from build123d import *

# Parameters (mm, degrees)
BOSS_EXTRUDE1_DEPTH     = 23
BOSS_EXTRUDE2_DEPTH     = 3
CUT_EXTRUDE1_DEPTH      = 143.828568571
CUT_EXTRUDE1_DEPTH_BACK = 143.828568571
SKETCH4_R               = 1.6
CUT_EXTRUDE2_DEPTH      = 1.5
SKETCH6_W               = 75
SKETCH6_H               = 20
CUT_EXTRUDE4_DEPTH      = 5
SKETCH8_R               = 1.25
SKETCH8_W               = 31.4
SKETCH8_H               = 20
CUT_EXTRUDE5_DEPTH      = 5
SKETCH9_W               = 2
SKETCH9_H               = 4.5
BOSS_EXTRUDE3_DEPTH     = 10
FILLET2_R               = 1
SKETCH10_W              = 12.12
SKETCH10_H              = 31
BOSS_EXTRUDE4_DEPTH     = 2.6
FILLET3_R               = 2
FILLET5_R               = 2
SKETCH11_W              = 2
SKETCH11_H              = 24
BOSS_EXTRUDE5_DEPTH     = 4
FILLET6_R               = 1
FILLET7_R               = 1
SKETCH12_W              = 10.12
SKETCH12_H              = 2
BOSS_EXTRUDE6_DEPTH     = 0.75
FILLET3_OF_MIRROR1_R    = 2
FILLET5_OF_MIRROR1_R    = 2
FILLET6_OF_MIRROR1_R    = 1
FILLET7_OF_MIRROR1_R    = 1


with BuildPart() as part:
    # Sketch1 → Boss-Extrude1 (new body)
    with BuildSketch(Plane(origin=(0, 0, 0), x_dir=(1, 0, 0), z_dir=(0, 1, 0))):
        with BuildLine():
            Line((12.5, 0), (87.5, 0))
            ThreePointArc((87.5, 0), (96.338834765, 3.661165235), (100, 12.5))
            Line((100, 12.5), (100, 87.5))
            ThreePointArc((100, 87.5), (96.338834765, 96.338834765), (87.5, 100))
            Line((87.5, 100), (12.5, 100))
            ThreePointArc((12.5, 100), (3.661165235, 96.338834765), (0, 87.5))
            Line((0, 87.5), (0, 12.5))
            ThreePointArc((0, 12.5), (3.661165235, 3.661165235), (12.5, 0))
        make_face()
        with BuildLine():
            Line((15, 97.5), (85, 97.5))
            ThreePointArc((85, 97.5), (93.838834765, 93.838834765), (97.5, 85))
            Line((97.5, 85), (97.5, 15))
            ThreePointArc((97.5, 15), (93.838834765, 6.161165235), (85, 2.5))
            Line((85, 2.5), (15, 2.5))
            ThreePointArc((15, 2.5), (6.161165235, 6.161165235), (2.5, 15))
            Line((2.5, 15), (2.5, 85))
            ThreePointArc((2.5, 85), (6.161165235, 93.838834765), (15, 97.5))
        make_face(mode=Mode.SUBTRACT)
    extrude(amount=BOSS_EXTRUDE1_DEPTH)

    # Sketch1<2> → Boss-Extrude2 (add)
    with BuildSketch(Plane(origin=(0, 0, 0), x_dir=(1, 0, 0), z_dir=(0, 1, 0))):
        with BuildLine():
            Line((15, 97.5), (85, 97.5))
            ThreePointArc((85, 97.5), (93.838834765, 93.838834765), (97.5, 85))
            Line((97.5, 85), (97.5, 15))
            ThreePointArc((97.5, 15), (93.838834765, 6.161165235), (85, 2.5))
            Line((85, 2.5), (15, 2.5))
            ThreePointArc((15, 2.5), (6.161165235, 6.161165235), (2.5, 15))
            Line((2.5, 15), (2.5, 85))
            ThreePointArc((2.5, 85), (6.161165235, 93.838834765), (15, 97.5))
        make_face()
    extrude(amount=BOSS_EXTRUDE2_DEPTH)

    # Sketch4 → Cut-Extrude1 (cut, two sides: drawn at the far end of the back side and taken through both)
    with BuildSketch(Plane(origin=(0, 3, 0), x_dir=(1, 0, 0), z_dir=(0, 1, 0)).offset(-CUT_EXTRUDE1_DEPTH_BACK)):
        with Locations(Location((88.890872965, 11.109127035, 0), (0, 0, 270))):
            Circle(SKETCH4_R)
        with Locations(Location((11.109127035, 88.890872965, 0), (0, 0, 270))):
            Circle(SKETCH4_R)
    extrude(amount=CUT_EXTRUDE1_DEPTH + CUT_EXTRUDE1_DEPTH_BACK, mode=Mode.SUBTRACT)

    # Sketch5 → Cut-Extrude2 (cut)
    with BuildSketch(Plane(origin=(0, 3, 0), x_dir=(1, 0, 0), z_dir=(0, 1, 0))):
        with BuildLine():
            Line((82.5, 4), (12.5, 4))
            ThreePointArc((12.5, 4), (8.964466094, 5.464466094), (7.5, 9))
            Line((7.5, 9), (7.5, 44))
            Line((7.5, 44), (82.5, 44))
            Line((82.5, 44), (82.5, 4))
        make_face()
    extrude(amount=-CUT_EXTRUDE2_DEPTH, mode=Mode.SUBTRACT)

    # Sketch6 → Cut-Extrude4 (cut)
    with BuildSketch(Plane.XY):
        with Locations((50, 13)):
            Rectangle(SKETCH6_W, SKETCH6_H)
    extrude(amount=-CUT_EXTRUDE4_DEPTH, mode=Mode.SUBTRACT)

    # Sketch8 → Cut-Extrude5 (cut)
    with BuildSketch(Plane(origin=(100, 0, 0), x_dir=(0, 0, -1), z_dir=(1, 0, 0))):
        with Locations((15.15, 11.76333723)):
            Circle(SKETCH8_R)
        with Locations(Location((51.25, 11.76333723, 0), (0, 0, 180))):
            Circle(SKETCH8_R)
        with Locations((33.2, 13)):
            Rectangle(SKETCH8_W, SKETCH8_H)
    extrude(amount=-CUT_EXTRUDE5_DEPTH, mode=Mode.SUBTRACT)

    # Sketch9 → Boss-Extrude3 (add)
    with BuildSketch(Plane.ZY):
        with Locations((-56.5, 11.5)):
            Rectangle(SKETCH9_W, SKETCH9_H)
    extrude(amount=BOSS_EXTRUDE3_DEPTH)

    # Fillet2
    fillet2_edges = [part.edges().sort_by_distance(p)[0] for p in [
        (0, 11.5, -57.5),
        (-5, 13.75, -57.5),
        (0, 9.25, -56.5),
        (-5, 9.25, -57.5),
        (0, 11.5, -55.5),
        (-5, 9.25, -55.5),
        (0, 13.75, -56.5),
        (-5, 13.75, -55.5),
        (-10, 11.5, -57.5),
        (-10, 9.25, -56.5),
        (-10, 11.5, -55.5),
        (-10, 13.75, -56.5),
    ]]
    fillet(fillet2_edges, radius=FILLET2_R - 0.0001)  # a hair under: the kernel refuses the full size

    # Sketch10 → Boss-Extrude4 (add)
    with BuildSketch(Plane(origin=(0, 0, 0), x_dir=(1, 0, 0), z_dir=(0, 1, 0))):
        with Locations((-6.06, 70)):
            Rectangle(SKETCH10_W, SKETCH10_H)
    boss_extrude4 = extrude(amount=BOSS_EXTRUDE4_DEPTH)

    # Fillet3
    fillet3_edges = [part.edges().sort_by_distance(p)[0] for p in [
        (0, 1.3, -54.5),
    ]]
    fillet(fillet3_edges, radius=FILLET3_R)

    # Fillet5
    fillet5_edges = [part.edges().sort_by_distance(p)[0] for p in [
        (0, 1.3, -85.5),
    ]]
    fillet(fillet5_edges, radius=FILLET5_R - 0.0001)  # a hair under: the kernel refuses the full size

    # Sketch11 → Boss-Extrude5 (add)
    with BuildSketch(Plane(origin=(0, 2.6, 0), x_dir=(1, 0, 0), z_dir=(0, 1, 0))):
        with Locations((-11.12, 73.5)):
            Rectangle(SKETCH11_W, SKETCH11_H)
    boss_extrude5 = extrude(amount=BOSS_EXTRUDE5_DEPTH)

    # Fillet6
    fillet6_edges = [part.edges().sort_by_distance(p)[0] for p in [
        (-12.12, 6.6, -73.5),
    ]]
    fillet(fillet6_edges, radius=FILLET6_R)

    # Fillet7
    fillet7_edges = [part.edges().sort_by_distance(p)[0] for p in [
        (-10.12, 2.6, -73.5),
    ]]
    fillet(fillet7_edges, radius=FILLET7_R)

    # Sketch12 → Boss-Extrude6 (add)
    with BuildSketch(Plane(origin=(0, 2.6, 0), x_dir=(1, 0, 0), z_dir=(0, 1, 0))):
        with Locations((-7.06, 55.5)):
            Rectangle(SKETCH12_W, SKETCH12_H)
    boss_extrude6 = extrude(amount=BOSS_EXTRUDE6_DEPTH)

    # Mirror1: Boss-Extrude4, Boss-Extrude5, Boss-Extrude6 across plane
    add(boss_extrude4.mirror(Plane.ZX.offset(11.5)))
    add(boss_extrude5.mirror(Plane.ZX.offset(11.5)))
    add(boss_extrude6.mirror(Plane.ZX.offset(11.5)))

    # Fillet3 of Mirror1
    fillet3_of_mirror1_edges = [part.edges().sort_by_distance(p)[0] for p in [
        (0, 21.7, -54.5),
    ]]
    fillet(fillet3_of_mirror1_edges, radius=FILLET3_OF_MIRROR1_R)

    # Fillet5 of Mirror1
    fillet5_of_mirror1_edges = [part.edges().sort_by_distance(p)[0] for p in [
        (0, 21.7, -85.5),
    ]]
    fillet(fillet5_of_mirror1_edges, radius=FILLET5_OF_MIRROR1_R - 0.0001)  # a hair under: the kernel refuses the full size

    # Fillet6 of Mirror1
    fillet6_of_mirror1_edges = [part.edges().sort_by_distance(p)[0] for p in [
        (-12.12, 16.4, -73.5),
    ]]
    fillet(fillet6_of_mirror1_edges, radius=FILLET6_OF_MIRROR1_R)

    # Fillet7 of Mirror1
    fillet7_of_mirror1_edges = [part.edges().sort_by_distance(p)[0] for p in [
        (-10.12, 20.4, -73.5),
    ]]
    fillet(fillet7_of_mirror1_edges, radius=FILLET7_OF_MIRROR1_R)


solid = part.part
Check sheet for the modelled part. Datum: model origin and axes. Units: mm. A direction names the side the tool comes from. Coordinates: 2 decimals unless noted, no trailing zeros. Write each loop counter-clockwise with the first axis right and the second up, starting at its lowest first coordinate (ties: lowest second). Pieces come first, ordered by that corner, then holes.
Item 1: Access from +Z, -Z, +X, -X, +Y, -Y to the whole of each face (thin tool, end or side, straight path). Record for faces 1 (the face through (-10.12, 5, -73)), 2 (the face through (-8, 2, -85.5)), 3 (the face through (87.5, 13, -1)), 4 (the face through (-11, 5, -61.5)).
Numbers:
face 1: +Z, -Z
face 2: -Z, -X, +Y, -Y
face 3: +Z, +Y
face 4: -X
Item 2: Depth check by flat-ended pin: pin 1 Ø2.5 at (x, y) = (-11, 4.5) entering from +Z; pin 2 Ø2 at (x, y) = (98, 14) entering from +Z; pin 3 Ø1 at (y, z) = (3, -10.5) entering from +X. Enter the tip coordinate at first touch or a pass-through.
Numbers:
pin 1: stops at z = -54.5
pin 2: stops at z = -4.38
pin 3: stops at x = 99.91
Item 3: Cross-section at A-A on z = -51.25. Record the boundary of the cut face in (x, y).
Numbers:
outline: (0, 0) - (100, 0) - (100, 10.51) - (97.5, 10.51) - (97.5, 3) - (2.5, 3) - (2.5, 23) - (0, 23) - close; (97.5, 13.01) - (100, 13.01) - (100, 23) - (97.5, 23) - close
Item 4: Scan lines: probe 1 along X at (y, z) = (2.5, -11); probe 2 along X at (y, z) = (8.25, -49.5); probe 3 along Y at (x, z) = (98, -51). Record each from-to range of solid material in increasing order.
Numbers:
probe 1: x = 0.09 to 7.5, 82.5 to 87.29, 90.49 to 99.91
probe 2: x = 0 to 2.5, 97.5 to 100
probe 3: y = 0 to 10.54, 12.99 to 23
Item 5: Cross-section at B-B on z = -75. Record the boundary of the cut face in (x, y).
Numbers:
outline: (-12.12, 0) - (100, 0) - (100, 23) - (97.5, 23) - (97.5, 3) - (2.5, 3) - (2.5, 23) - (-12.12, 23) - (-12.12, 17.4) arc R1 ccw to (-11.12, 16.4) - (-10.12, 16.4) - (-10.12, 19.4) arc R1 cw to (-9.12, 20.4) - (0, 20.4) - (0, 2.6) - (-9.12, 2.6) arc R1 cw to (-10.12, 3.6) - (-10.12, 6.6) - (-11.12, 6.6) arc R1 ccw to (-12.12, 5.6) - close
Item 6: Mould release check, pull along Y, two halves, no side actions. Record for faces 5 (the face through (0, 11, -51)), 6 (the face through (45, 0, -51)), 7 (the face through (50, 13, -97.5)): released by +Y, released by -Y, zero draft, split by the parting line, or undercut.
Numbers:
face 5: undercut
face 6: released by -Y
face 7: zero draft
